```python
from build123d import *

# Parameters (mm, degrees)
ESBO_O1_W                = 80
ESBO_O1_H                = 65
RESSALTO_EXTRUS_O1_DEPTH = 13
ESBO_O3_W                = 13
ESBO_O3_H                = 65
RESSALTO_EXTRUS_O2_DEPTH = 6.5
CORTE_EXTRUS_O1_DEPTH    = 65
CORTE_EXTRUS_O2_REACH    = 110.978
ESBO_O5_W                = 10
ESBO_O5_H                = 45
RESSALTO_EXTRUS_O4_DEPTH = 2.5
ESBO_O7_W                = 16.5
ESBO_O7_H                = 10
RESSALTO_EXTRUS_O5_DEPTH = 2.5
ESBO_O9_R                = 1.25
CORTE_EXTRUS_O3_DEPTH    = 129.092983805
ESBO_O11_W               = 14
ESBO_O11_H               = 10
CORTE_EXTRUS_O4_DEPTH    = 0.3


with BuildPart() as part:
    # Esboço1 → Ressalto-extrusão1 (new body)
    with BuildSketch(Plane.XY):
        with Locations((40, 32.5)):
            Rectangle(ESBO_O1_W, ESBO_O1_H)
    extrude(amount=RESSALTO_EXTRUS_O1_DEPTH)

    # Esboço3 → Ressalto-extrusão2 (add)
    with BuildSketch(Plane.ZY):
        with Locations((6.5, 32.5)):
            Rectangle(ESBO_O3_W, ESBO_O3_H)
    extrude(amount=RESSALTO_EXTRUS_O2_DEPTH)

    # Esboço4 → Corte-extrusão1 (cut)
    with BuildSketch(Plane(origin=(0, 0, 0), x_dir=(-1, 0, 0), z_dir=(0, -1, 0))):
        with BuildLine():
            ThreePointArc((-14.5, -13), (-5.25, -22.25), (4, -13))
            Line((4, -13), (-5.25, -13))
            Line((-5.25, -13), (-14.5, -13))
        make_face()
        with BuildLine():
            Line((-5.25, -13), (4, -13))
            ThreePointArc((4, -13), (-5.25, -3.75), (-14.5, -13))
            Line((-14.5, -13), (-5.25, -13))
        make_face()
        with BuildLine():
            ThreePointArc((-35, -13), (-25.75, -22.25), (-16.5, -13))
            Line((-16.5, -13), (-25.75, -13))
            Line((-25.75, -13), (-35, -13))
        make_face()
        with BuildLine():
            Line((-25.75, -13), (-16.5, -13))
            ThreePointArc((-16.5, -13), (-25.75, -3.75), (-35, -13))
            Line((-35, -13), (-25.75, -13))
        make_face()
        with BuildLine():
            ThreePointArc((-56, -13), (-46.75, -22.25), (-37.5, -13))
            Line((-37.5, -13), (-46.75, -13))
            Line((-46.75, -13), (-56, -13))
        make_face()
        with BuildLine():
            Line((-46.75, -13), (-37.5, -13))
            ThreePointArc((-37.5, -13), (-46.75, -3.75), (-56, -13))
            Line((-56, -13), (-46.75, -13))
        make_face()
        with BuildLine():
            ThreePointArc((-77, -13), (-67.75, -22.25), (-58.5, -13))
            Line((-58.5, -13), (-67.75, -13))
            Line((-67.75, -13), (-77, -13))
        make_face()
        with BuildLine():
            Line((-67.75, -13), (-58.5, -13))
            ThreePointArc((-58.5, -13), (-67.75, -3.75), (-77, -13))
            Line((-77, -13), (-67.75, -13))
        make_face()
    extrude(amount=-CORTE_EXTRUS_O1_DEPTH, mode=Mode.SUBTRACT)

    # Esboço5 → Corte-extrusão2 (cut, up to next)
    with BuildSketch(Plane(origin=(80, 0, 0), x_dir=(0, 0, -1), z_dir=(1, 0, 0)), mode=Mode.PRIVATE) as corte_extrus_o2_sk1:
        with Locations((-8, 32.5)):
            Rectangle(ESBO_O5_W, ESBO_O5_H)
    corte_extrus_o2_tool1 = extrude(corte_extrus_o2_sk1.sketch, amount=-CORTE_EXTRUS_O2_REACH, mode=Mode.PRIVATE) & part.part
    add(corte_extrus_o2_tool1.solids().sort_by_distance((80, 32.5, 8))[0], mode=Mode.SUBTRACT)

    # Esboço6 → Ressalto-extrusão4 (add)
    with BuildSketch(Plane(origin=(80, 0, 0), x_dir=(0, 0, -1), z_dir=(1, 0, 0))):
        Polygon((6.25, -7.5), (6.25, 32.5), (6.25, 72.5), (-48.75, 72.5), (-48.75, -7.5), align=None)
    extrude(amount=RESSALTO_EXTRUS_O4_DEPTH)

    # Esboço7 → Ressalto-extrusão5 (add)
    with BuildSketch(Plane(origin=(0, 72.5, 0), x_dir=(1, 0, 0), z_dir=(0, 1, 0))):
        with Locations((74.25, -23.75)):
            Rectangle(ESBO_O7_W, ESBO_O7_H)
    ressalto_extrus_o5 = extrude(amount=RESSALTO_EXTRUS_O5_DEPTH)

    # Espelhar1: Ressalto-extrusão5 across plane
    add(ressalto_extrus_o5.mirror(Plane(origin=(0, 32.5, 0), x_dir=(0, 0, 1), z_dir=(0, -1, 0))))

    # Esboço9 → Corte-extrusão3 (cut, through all)
    with BuildSketch(Plane(origin=(0, 75, 0), x_dir=(1, 0, 0), z_dir=(0, 1, 0))):
        with Locations(Location((71, -23.75, 0), (0, 0, 270))):
            Circle(ESBO_O9_R)
    extrude(amount=-CORTE_EXTRUS_O3_DEPTH, mode=Mode.SUBTRACT)

    # Esboço11 → Corte-extrusão4 (cut)
    with BuildSketch(Plane.XZ.offset(-72.5)):
        with Locations((73, 23.75)):
            Rectangle(ESBO_O11_W, ESBO_O11_H)
    corte_extrus_o4 = extrude(amount=-CORTE_EXTRUS_O4_DEPTH, mode=Mode.SUBTRACT)

    # Espelhar2: Corte-extrusão4 across plane
    add(corte_extrus_o4.mirror(Plane(origin=(0, 32.5, 0), x_dir=(0, 0, 1), z_dir=(0, -1, 0))), mode=Mode.SUBTRACT)


solid = part.part
```
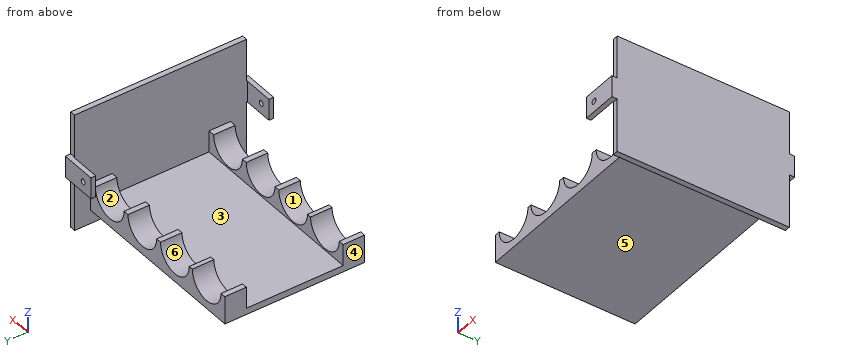
The model under review builds one solid part; all positions refer to its coordinate system, in mm. Face numbers are marked on the shaded views. A direction names the side the tool comes from. Round coordinates to 2 decimals unless told otherwise and drop trailing zeros. Loops run counter-clockwise (first coordinate to the right, second up) from the corner with the lowest first, then second, coordinate; pieces in that order, holes last. Notation, with made-up numbers: (27.5, 69.5) -> (76.5, 69.5) arc R28 ccw to (76.5, 92.5) -> close; hole circle Ø1 at (70, 21.25). An arc over 180 degrees is marked (long way). Answer in a Markdown table with one row per item.
1) Wall thickness on line 1 along Z through (x, y) = (71, 74.5); line 2 along X through (y, z) = (-8.4, 23.75); line 3 along Y through (x, z) = (21, 3.5): over which ranges is each line inside the solid? List them lowest first.
Taken from the geometry:
| item | result |
|---|---|
| line 1 | z = 18.75 to 22.5, 25 to 28.75 |
| line 2 | x = 66 to 69.75, 72.25 to 82.5 |
| line 3 | y = 0 to 10, 55 to 65 |
2) Consider section C-C, the plane y = 17. Write out the cut boundary in (x, z).
Taken from the geometry:
| item | result |
|---|---|
| outline | (-6.5, 0) -> (80, 0) -> (80, -6.25) -> (82.5, -6.25) -> (82.5, 48.75) -> (80, 48.75) -> (80, 3) -> (-6.5, 3) -> close |
3) Tool access review of the marked faces 5 and 6: name each direction out of +Z, -Z, +X, -X, +Y, -Y from which nothing blocks a thin tool from reaching the whole face with its end or side.
Taken from the geometry:
| item | result |
|---|---|
| face 5 | -Z, -X, +Y, -Y |
| face 6 | +Z, +Y, -Y |
4) Consider section B-B, the plane z = 23.75. Write out the cut boundary in (x, y).
Taken from the geometry:
| item | result |
|---|---|
| outline | (66, -10) -> (69.75, -10) -> (69.75, -7.8) -> (66, -7.8) -> close; (66, 72.8) -> (69.75, 72.8) -> (69.75, 75) -> (66, 75) -> close; (72.25, -10) -> (82.5, -10) -> (82.5, 75) -> (72.25, 75) -> (72.25, 72.8) -> (80, 72.8) -> (80, -7.8) -> (72.25, -7.8) -> close |
5) Consider section A-A, the plane x = 67.75. Write out the cut boundary in (y, z).
Taken from the geometry:
| item | result |
|---|---|
| outline | (-10, 18.75) -> (-7.8, 18.75) -> (-7.8, 28.75) -> (-10, 28.75) -> close; (0, 0) -> (65, 0) -> (65, 3.75) -> (55, 3.75) -> (55, 3) -> (10, 3) -> (10, 3.75) -> (0, 3.75) -> close; (72.8, 18.75) -> (75, 18.75) -> (75, 28.75) -> (72.8, 28.75) -> close |
6) For pin 1 Ø5 at (x, z) = (54, 8) entering from -Y; pin 2 Ø2.5 at (y, z) = (-9.5, 25.5) entering from -X; pin 3 Ø1.5 at (x, z) = (22, 1) entering from +Y, all flat-tipped, find the tip position at first contact; note any pin that passes through.
Taken from the geometry:
| item | result |
|---|---|
| pin 1 | stops at y = 0 |
| pin 2 | stops at x = 66 |
| pin 3 | stops at y = 65 |
7) Draft analysis for pull direction X (two halves, no side actions). For the marked faces 1, 2, 3 and 4, state which applies: pulls with the +X half, pulls with the -X half, needs draft (parallel to the pull), parting line crosses it, or undercut.
Taken from the geometry:
| item | result |
|---|---|
| face 1 | undercut |
| face 2 | undercut |
| face 3 | needs draft |
| face 4 | pulls with the -X half |
8) Consider section D-D, the plane x = 25.75. Write out the cut boundary in (y, z).
Taken from the geometry:
| item | result |
|---|---|
| outline | (0, 0) -> (65, 0) -> (65, 3.75) -> (55, 3.75) -> (55, 3) -> (10, 3) -> (10, 3.75) -> (0, 3.75) -> close |
